CAD build for the part. Positions are in the model's coordinates, mm. A direction names the side the tool comes from. Round coordinates to 2 decimals unless told otherwise and drop trailing zeros. Loops run counter-clockwise (first coordinate to the right, second up) from the corner with the lowest first, then second, coordinate; pieces in that order, holes last. Notation, with made-up numbers: M 71,64 L 105,64 A32 ccw 105,94 Z; hole C -29,33.5 d6. An arc over 180 degrees is marked long. Use a Markdown table: item, result. Add a question column.
(1) Wall check: L1, parallel to Y at x = 0, z = -54; L2, parallel to Y at x = 23, z = -2; L3, parallel to Z at x = 6.5, y = -24. Give the ranges that are in metal, low to high.
(2) Two-plate mould, pull along Y, no slides. Class faces 4 (the face through (27.436, 27.47, -2.504)), 5 (the face through (19.914, -20.072, -29.874)), 6 (the face through (0.661, 5.037, -54.12)): released by +Y, released by -Y, zero draft, split by the parting line, or undercut.
(3) Band-saw the part on D-D, the plane z = -11.5. Write the cut outline in (x, y), and give its area (3 significant figures).
(4) Flat gauge pins, fed straight in: P1, Ø6.5, axis at x = 23.505, y = -23.876, coming from the +Z side; P2, Ø8, axis at x = -23.495, y = -23.876, coming from the -Z side; P3, Ø3, axis at y = -29.5, z = -48.5, coming from the -X side. Where does each tip first touch, or does it go through?
(5) Which spindle directions (+Z, -Z, +X, -X, +Y, -Y) get a long thin tool onto all of the face, cutting with end or side? Do faces 1 (the face through (0, -29, -51.562)), 2 (the face through (-20.076, -19.91, -29.874)), 3 (the face through (-2.222, -29, -49)). Say none if no direction does.
(6) Band-saw the part on B-B, the plane z = -48.5. Write the cut outline in (x, y).
from build123d import *

# Parameters (mm, degrees)
BOSS_EXTRUDE1_DEPTH = 5.08
SKETCH2_R           = 2.5
SKETCH2_R_2         = 2.54
CUT_EXTRUDE1_DEPTH  = 12.7
SKETCH3_R           = 3.175
BOSS_EXTRUDE2_DEPTH = 20
BOSS_EXTRUDE3_DEPTH = 50.292
SKETCH7_R           = 5.08
CUT_EXTRUDE2_DEPTH  = 2.54
SKETCH8_W           = 4.445
SKETCH8_H           = 4.445
BOSS_EXTRUDE4_DEPTH = 2.54
SKETCH9_R           = 18.923
BOSS_EXTRUDE5_DEPTH = 1.27


with BuildPart() as part:
    # Sketch1 → Boss-Extrude1 (new body)
    with BuildSketch(Plane.XY):
        with BuildLine():
            Line((-25.66, 28.194), (25.66, 28.194))
            ThreePointArc((25.66, 28.194), (27.456051224, 27.450051224), (28.2, 25.654))
            Line((28.2, 25.654), (28.2, -25.654))
            ThreePointArc((28.2, -25.654), (27.456051224, -27.450051224), (25.66, -28.194))
            Line((25.66, -28.194), (-25.66, -28.194))
            ThreePointArc((-25.66, -28.194), (-27.456051224, -27.450051224), (-28.2, -25.654))
            Line((-28.2, -25.654), (-28.2, 25.654))
            ThreePointArc((-28.2, 25.654), (-27.456051224, 27.450051224), (-25.66, 28.194))
        make_face()
    extrude(amount=-BOSS_EXTRUDE1_DEPTH)

    # Sketch2 → Cut-Extrude1 (cut)
    with BuildSketch(Plane.XY):
        with Locations((-23.495, 23.876)):
            Circle(SKETCH2_R)
        with Locations((23.505, 23.876)):
            Circle(SKETCH2_R_2)
        with Locations((-23.495, -23.876)):
            Circle(SKETCH2_R_2)
        with Locations((23.505, -23.876)):
            Circle(SKETCH2_R_2)
    extrude(amount=-CUT_EXTRUDE1_DEPTH, mode=Mode.SUBTRACT)

    # Sketch3 → Boss-Extrude2 (add)
    with BuildSketch(Plane.XY):
        Circle(SKETCH3_R)
    extrude(amount=BOSS_EXTRUDE2_DEPTH)

    # Sketch6 → Boss-Extrude3 (add)
    with BuildSketch(Plane(origin=(0, 0, -5.08), x_dir=(-1, 0, 0), z_dir=(0, 0, -1))):
        with BuildLine():
            Line((-15.620607632, 28.193981005), (15.620607632, 28.193981005))
            ThreePointArc((15.620607632, 28.193981005), (16.309436696, 27.924821363), (16.633295319, 27.25995447))
            ThreePointArc((16.633295319, 27.25995447), (19.995115916, 19.990526597), (27.265660549, 16.631121879))
            ThreePointArc((27.265660549, 16.631121879), (27.930749509, 16.307360153), (28.200023614, 15.618407008))
            Line((28.200023614, 15.618407008), (28.200023614, -15.618407008))
            ThreePointArc((28.200023614, -15.618407008), (27.930742821, -16.307367402), (27.265640888, -16.631123464))
            ThreePointArc((27.265640888, -16.631123464), (19.994877492, -19.99046435), (16.632859418, -27.259990196))
            ThreePointArc((16.632859418, -27.259990196), (16.308995981, -27.924846048), (15.620173086, -28.194))
            Line((15.620173086, -28.194), (-15.620173086, -28.194))
            ThreePointArc((-15.620173086, -28.194), (-16.308986965, -27.924854363), (-16.632857438, -27.260014646))
            ThreePointArc((-16.632857438, -27.260014646), (-19.994954858, -19.990760744), (-27.265596467, -16.631665336))
            ThreePointArc((-27.265596467, -16.631665336), (-27.93071213, -16.307915269), (-28.2, -15.618947204))
            Line((-28.2, -15.618947204), (-28.2, 15.618947204))
            ThreePointArc((-28.2, 15.618947204), (-27.930718818, 16.30790802), (-27.265616128, 16.631663752))
            ThreePointArc((-27.265616128, 16.631663752), (-19.995193282, 19.990822991), (-16.633293339, 27.25997892))
            ThreePointArc((-16.633293339, 27.25997892), (-16.30942768, 27.924829678), (-15.620607632, 28.193981005))
        make_face()
    extrude(amount=BOSS_EXTRUDE3_DEPTH)

    # Sketch7 → Cut-Extrude2 (cut)
    with BuildSketch(Plane(origin=(0, 0, -55.372), x_dir=(-1, 0, 0), z_dir=(0, 0, -1))):
        Circle(SKETCH7_R)
    extrude(amount=-CUT_EXTRUDE2_DEPTH, mode=Mode.SUBTRACT)

    # Sketch8 → Boss-Extrude4 (add)
    with BuildSketch(Plane(origin=(0, -28.194, 0), x_dir=(-1, 0, 0), z_dir=(0, -1, 0))):
        with Locations((0, 49.3395)):
            Rectangle(SKETCH8_W, SKETCH8_H)
    extrude(amount=BOSS_EXTRUDE4_DEPTH)

    # Sketch9 → Boss-Extrude5 (add)
    with BuildSketch(Plane.XY):
        Circle(SKETCH9_R)
    extrude(amount=BOSS_EXTRUDE5_DEPTH)


solid = part.part
Return value:
| question | item | result |
|---|---|---|
| 1 | L1 | -28.19 to -5.08, 5.08 to 28.19 |
| 1 | L2 | -28.19 to -26.37, -21.39 to 21.39, 26.37 to 28.19 |
| 1 | L3 | -55.37 to 0 |
| 2 | face 4 | released by +Y |
| 2 | face 5 | released by -Y |
| 2 | face 6 | undercut |
| 3 | outline | M -28.2,-15.62 A1.02 ccw -27.27,-16.63 A11.6 cw -16.63,-27.26 A1.02 ccw -15.62,-28.19 L 15.62,-28.19 A1.02 ccw 16.63,-27.26 A11.6 cw 27.27,-16.63 A1.02 ccw 28.2,-15.62 L 28.2,15.62 A1.02 ccw 27.27,16.63 A11.6 cw 16.63,27.26 A1.02 ccw 15.62,28.19 L -15.62,28.19 A1.02 ccw -16.63,27.26 A11.6 cw -27.27,16.63 A1.02 ccw -28.2,15.62 Z |
| 3 | area | 2,760 mm^2 |
| 4 | P1 | z = 0 |
| 4 | P2 | z = -5.08 |
| 4 | P3 | x = -16.22 |
| 5 | face 1 | -Z, +X, -X, -Y |
| 5 | face 2 | -Z, -X, -Y |
| 5 | face 3 | +Z, -Z, -X, -Y |
| 6 | outline | M -28.2,-15.62 A1.02 ccw -27.27,-16.63 A11.6 cw -16.63,-27.26 A1.02 ccw -15.62,-28.19 L -2.22,-28.19 L -2.22,-30.73 L 2.22,-30.73 L 2.22,-28.19 L 15.62,-28.19 A1.02 ccw 16.63,-27.26 A11.6 cw 27.27,-16.63 A1.02 ccw 28.2,-15.62 L 28.2,15.62 A1.02 ccw 27.27,16.63 A11.6 cw 16.63,27.26 A1.02 ccw 15.62,28.19 L -15.62,28.19 A1.02 ccw -16.63,27.26 A11.6 cw -27.27,16.63 A1.02 ccw -28.2,15.62 Z |
